Source: CAD feature listing. Evaluate the final solid. Frame: model axes, mm. A direction names the side the tool comes from. Give positions to 0.01 mm unless a question says otherwise; leave off trailing zeros. Order: outer loops, then holes, each group sorted by start corner. A loop starts at its lowest first (then second) coordinate and runs counter-clockwise, first axis right, second up.
1) Section A-A, the plane z = 7.5. Return loops of the section in (x, y) (3 decimals).
2) Draft query along X for faces 4 (the face through (0, 6, 6)), 5 (the face through (7.28, 0.99, 9.21)), 6 (the face through (7, 13, 15)). Return one class per face: released by +X, released by -X, zero draft, split by the parting line, or undercut.
3) First-contact query: P1, Ø3, axis at x = 7.5, y = 7.5, coming from the -Z side; P2, Ø5.5, axis at x = 7, z = 7, coming from the +Y side; P3, Ø8, axis at y = 7.5, z = 7.5, coming from the +X side. Flat tips, straight axial feed; report the tip coordinate or a pass-through.
4) Material intervals for line 1 (Z direction, x = 1.35, y = 7.5) (3 decimals); line 2 (Z direction, x = 14.45, y = 7.5), sorted ascending.
5) Section D-D, the plane y = 12.25. Return loops of the section in (x, z).
6) Section B-B, the plane y = 7.5. Return loops of the section in (x, z) (3 decimals), plus the area to 3 significant figures.
7) Access query for faces 1 (the face through (6, 2, 6)), 2 (the face through (7.28, 5.79, 0.89)), 3 (the face through (2.73, 14.01, 9)). Directions: +Z, -Z, +X, -X, +Y, -Y. A direction counts if a zero-diameter tool reaches every point of the face in a straight line with its end or side. Return the directions, or none.
```python
from build123d import *

# Parameters (mm, degrees)
F0_W      = 15
F0_H      = 15
F1_DEPTH  = 15
F2_W      = 11
F2_H      = 11
F3_DEPTH  = 11
F6_R      = 1.725
F7_DEPTH  = 2
F8_R      = 1.725
F9_DEPTH  = 2
F10_R     = 1.725
F11_DEPTH = 2
F12_R     = 5
F13_DEPTH = 7.5
F14_R     = 5
F15_DEPTH = 7.5
F16_R     = 5
F17_DEPTH = 7.5
F18_R     = 3.5
F19_DEPTH = 13
F20_R     = 3.5
F21_DEPTH = 13
F22_R     = 3.5
F23_DEPTH = 13
F24_R     = 1.725
F25_DEPTH = 0.2


with BuildPart() as f1:
    # F0 (on Top) → F1 (new body)
    with BuildSketch(Plane.XY):
        with Locations((7.5, 7.5)):
            Rectangle(F0_W, F0_H)
    extrude(amount=F1_DEPTH)


with BuildPart() as f3:
    # F2 (on Top) → F3 (new body)
    with BuildSketch(Plane.XY):
        with Locations((7.5, 7.5)):
            Rectangle(F2_W, F2_H)
    extrude(amount=F3_DEPTH)


with BuildPart() as f3_1:
    # F4: moved
    add(f3.part.moved(Location((0, 0, 2))))


with BuildPart() as f1_1:
    add(f1.part)

    # F5: cut F3
    add(f3_1.part, mode=Mode.SUBTRACT)

    # F6 (on face) → F7 (cut, through all)
    with BuildSketch(Plane.XZ):
        with Locations((7.5, 7.5)):
            Circle(F6_R)
    extrude(amount=-F7_DEPTH, mode=Mode.SUBTRACT)

    # F8 (on face) → F9 (cut, through all)
    with BuildSketch(Plane(origin=(0, 0, 0), x_dir=(0, -1, 0), z_dir=(-1, 0, 0))):
        with Locations((-7.5, 7.5)):
            Circle(F8_R)
    extrude(amount=-F9_DEPTH, mode=Mode.SUBTRACT)

    # F10 (on face) → F11 (cut, through all)
    with BuildSketch(Plane(origin=(0, 0, 0), x_dir=(1, 0, 0), z_dir=(0, 0, -1))):
        with Locations((7.5, -7.5)):
            Circle(F10_R)
    extrude(amount=-F11_DEPTH, mode=Mode.SUBTRACT)

    # F12 (on face) → F13 (cut)
    with BuildSketch(Plane(origin=(0, 15, 0), x_dir=(-1, 0, 0), z_dir=(0, 1, 0))):
        with Locations((-7.5, 7.5)):
            Circle(F12_R)
    extrude(amount=-F13_DEPTH, mode=Mode.SUBTRACT)

    # F14 (on face) → F15 (cut)
    with BuildSketch(Plane.YZ.offset(15)):
        with Locations((7.5, 7.5)):
            Circle(F14_R)
    extrude(amount=-F15_DEPTH, mode=Mode.SUBTRACT)

    # F16 (on face) → F17 (cut)
    with BuildSketch(Plane.XY.offset(15)):
        with Locations((7.5, 7.5)):
            Circle(F16_R)
    extrude(amount=-F17_DEPTH, mode=Mode.SUBTRACT)

    # F18 (on face) → F19 (cut)
    with BuildSketch(Plane(origin=(0, 15, 0), x_dir=(-1, 0, 0), z_dir=(0, 1, 0))):
        with Locations((-7.5, 7.5)):
            Circle(F18_R)
    extrude(amount=-F19_DEPTH, mode=Mode.SUBTRACT)

    # F20 (on face) → F21 (cut)
    with BuildSketch(Plane.YZ.offset(15)):
        with Locations((7.5, 7.5)):
            Circle(F20_R)
    extrude(amount=-F21_DEPTH, mode=Mode.SUBTRACT)

    # F22 (on face) → F23 (cut)
    with BuildSketch(Plane.XY.offset(15)):
        with Locations((7.5, 7.5)):
            Circle(F22_R)
    extrude(amount=-F23_DEPTH, mode=Mode.SUBTRACT)

    # F24 (on face) → F25 (join)
    with BuildSketch(Plane.XY.offset(2)):
        with Locations((7.5, 7.5)):
            Circle(F24_R)
    extrude(amount=-F25_DEPTH)


solid = f1_1.part
```
From the geometry:
1. outline: (0, 0) - (5.775, 0) - (5.775, 2) - (2, 2) - (2, 5.775) - (0, 5.775) - close; (0, 9.225) - (2, 9.225) - (2, 13) - (2.5, 13) - (2.5, 15) - (0, 15) - close; (9.225, 0) - (15, 0) - (15, 2.5) - (13, 2.5) - (13, 2) - (9.225, 2) - close; (12.5, 13) - (13, 13) - (13, 12.5) - (15, 12.5) - (15, 15) - (12.5, 15) - close
2. face 4: released by -X
2. face 5: undercut
2. face 6: zero draft
3. P1: stops at z = 1.8
3. P2: stops at y = 2
3. P3: stops at x = 2
4. line 1: z = 0 to 5.775, 9.225 to 15
4. line 2: z = 0 to 2.5, 12.5 to 15
5. outline: (0, 0) - (15, 0) - (15, 5.94) - (13, 5.94) - (13, 2) - (2, 2) - (2, 13) - (5.94, 13) - (5.94, 15) - (0, 15) - close; (9.06, 13) - (13, 13) - (13, 9.06) - (15, 9.06) - (15, 15) - (9.06, 15) - close
6. outline: (0, 0) - (5.775, 0) - (5.775, 1.8) - (9.225, 1.8) - (9.225, 0) - (15, 0) - (15, 2.5) - (13, 2.5) - (13, 2) - (2, 2) - (2, 5.775) - (0, 5.775) - close; (0, 9.225) - (2, 9.225) - (2, 13) - (2.5, 13) - (2.5, 15) - (0, 15) - close; (12.5, 13) - (13, 13) - (13, 12.5) - (15, 12.5) - (15, 15) - (12.5, 15) - close
6. area: 50.9 mm2
7. face 1: none
7. face 2: -Z
7. face 3: +Y
